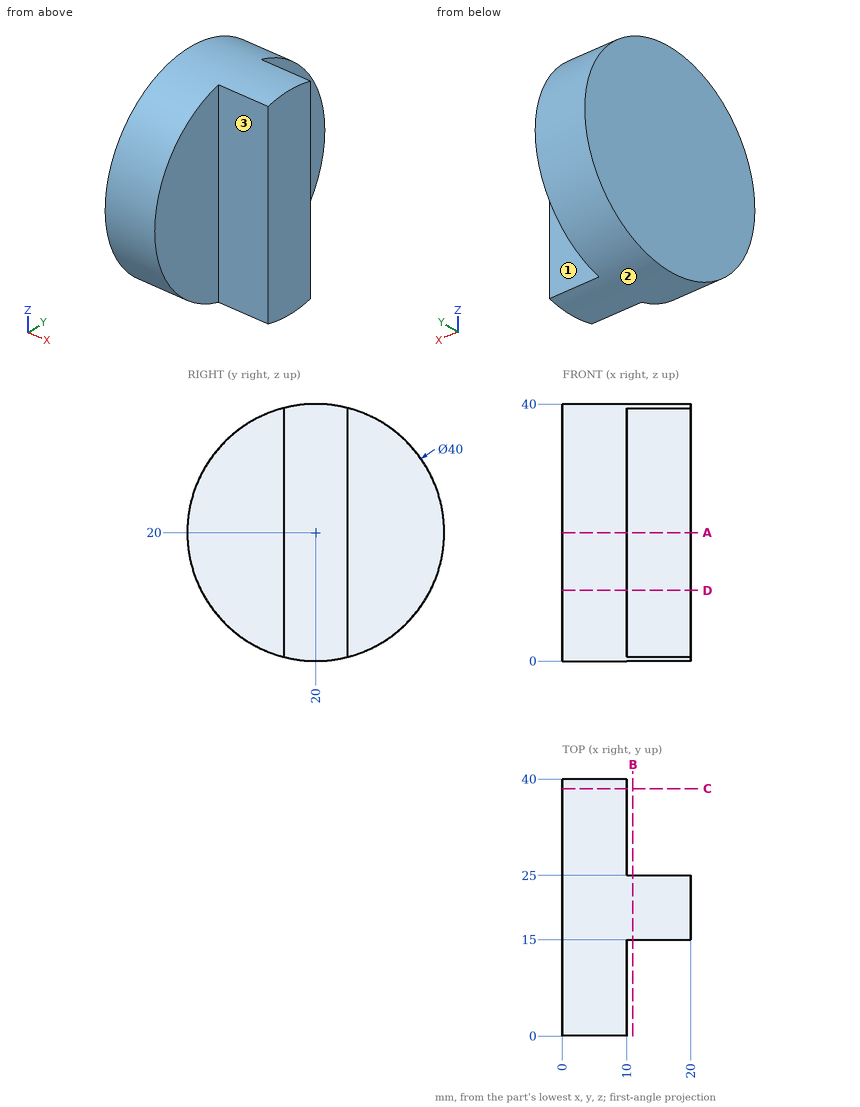
Here's the drawing with two shaded views (mm, measured from the low corner). I have some questions. A direction names the side the tool comes from. Give positions to 0.01 mm unless a question says otherwise; leave off trailing zeros. Order: outer loops, then holes, each group sorted by start corner. A loop starts at its lowest first (then second) coordinate and runs counter-clockwise, first axis right, second up. Notation, with made-up numbers: (-14, 74.25) -> (17, 74.25) arc R34 ccw to (17, 112.25) -> close; hole circle Ø4 at (39, 49). An arc over 180 degrees is marked (long way). Use a Markdown table: item, result. Add a question column.
Item 1: I need wall thicknesses on line 1 (Y direction, x = 11.75, z = 10.5); line 2 (X direction, y = 6, z = 15); line 3 (Z direction, x = 9, y = 34). Which ranges of each line are inside material? Lowest first, please.
Item 2: Will these pins go through, and if not, where does the flat tip stop? pin 1 (2 mm diameter, centred on x = 9.5, y = 8, fed in from -Z); pin 2 (3 mm diameter, centred on x = 12.5, z = 7, fed in from +Y); pin 3 (1.5 mm diameter, centred on x = 17, y = 24, fed in from +Z).
Item 3: For the marked faces 1, 2 and 3, which set-ups out of +Z, -Z, +X, -X, +Y, -Y let a thin tool reach every point of the face, with its end or its side?
Item 4: Imagine slicing it at A-A on z = 20. Please give me the cut outline in (x, y).
Item 5: Imagine slicing it at D-D on z = 11. Please give me the cut outline in (x, y), plus the area to 3 significant figures.
Item 6: Imagine slicing it at B-B on x = 11. Please give me the cut outline in (y, z), plus the area to 3 significant figures.
Item 7: Imagine slicing it at C-C on y = 38.5. Please give me the cut outline in (x, z), plus the area to 3 significant figures.
Data:
| question | item | result |
|---|---|---|
| 1 | line 1 | y = 15 to 25 |
| 1 | line 2 | x = 0 to 10 |
| 1 | line 3 | z = 5.72 to 34.28 |
| 2 | pin 1 | stops at z = 3.3 |
| 2 | pin 2 | stops at y = 25 |
| 2 | pin 3 | stops at z = 39.73 |
| 3 | face 1 | +Z, -Z, +X, +Y |
| 3 | face 2 | +X, -X |
| 3 | face 3 | +Z, -Z, +X, -Y |
| 4 | outline | (0, 0) -> (10, 0) -> (10, 15) -> (20, 15) -> (20, 25) -> (10, 25) -> (10, 40) -> (0, 40) -> close |
| 5 | outline | (0, 2.14) -> (10, 2.14) -> (10, 15) -> (20, 15) -> (20, 25) -> (10, 25) -> (10, 37.86) -> (0, 37.86) -> close |
| 5 | area | 457 mm² |
| 6 | outline | (15, 0.64) arc R20 ccw to (25, 0.64) -> (25, 39.36) arc R20 ccw to (15, 39.36) -> close |
| 6 | area | 396 mm² |
| 7 | outline | (0, 12.4) -> (10, 12.4) -> (10, 27.6) -> (0, 27.6) -> close |
| 7 | area | 152 mm² |
